```python
from build123d import *

# Parameters (mm, degrees)
SKETCH2_R           = 1.4
BOSS_EXTRUDE1_DEPTH = 2.5
SKETCH3_W           = 13
SKETCH3_H           = 4.686630076
BOSS_EXTRUDE3_DEPTH = 6
FILLET1_R           = 2
BOSS_EXTRUDE4_DEPTH = 0.5
CUT_EXTRUDE1_DEPTH  = 7


with BuildPart() as part:
    # Sketch1 → Revolve1 (revolve)
    with BuildSketch(Plane(origin=(0, 0, 0), x_dir=(0, 0, -1), z_dir=(1, 0, 0)), mode=Mode.PRIVATE) as revolve1_sk:
        Polygon((0, 0), (0, 11.5), (11, 11.5), (11, 4.5), (21, 4.5), (21, 3.175), (31, 3.175), (31, 0), align=None)
    revolve(revolve1_sk.sketch.rotate(Axis((0, 0, 0), (0, 0, -1)), 90), axis=Axis((0, 0, 0), (0, 0, -1)))

    # Sketch2 → Boss-Extrude1 (add)
    with BuildSketch(Plane(origin=(0, 0, -11), x_dir=(-1, 0, 0), z_dir=(0, 0, -1))):
        with Locations(Location((-10, 0, 0), (0, 0, 180))):
            Circle(SKETCH2_R)
    extrude(amount=BOSS_EXTRUDE1_DEPTH)

    # Sketch3 → Boss-Extrude3 (add)
    with BuildSketch(Plane(origin=(0, 0, -5), x_dir=(-1, 0, 0), z_dir=(0, 0, -1))):
        with Locations((0, -10.656684962)):
            Rectangle(SKETCH3_W, SKETCH3_H)
    extrude(amount=BOSS_EXTRUDE3_DEPTH)

    # Fillet1
    fillet1_edges = [part.edges().sort_by_distance(p)[0] for p in [
        (6.5, -9.486832981, -8),
        (-6.5, -9.486832981, -8),
    ]]
    fillet(fillet1_edges, radius=FILLET1_R)

    # Sketch4 → Boss-Extrude4 (add)
    # profile 1 of 3: a face of its own
    with BuildSketch(Plane(origin=(0, 0, -6), x_dir=(-1, 0, 0), z_dir=(0, 0, -1))):
        with BuildLine():
            Line((-5.420458078, -13), (-5.420458078, -13.616327338))
            Line((-5.420458078, -13.616327338), (-6, -13.616327338))
            Line((-6, -13.616327338), (-6, -15.080506085))
            Line((-6, -15.080506085), (-6.5, -15.080506085))
            Line((-6.5, -15.080506085), (-6.5, -18.5))
            ThreePointArc((-6.5, -18.5), (-5, -20), (-3.5, -18.5))
            Line((-3.5, -18.5), (-3.5, -15.080506085))
            Line((-3.5, -15.080506085), (-4, -15.080506085))
            Line((-4, -15.080506085), (-4, -13.616327338))
            Line((-4, -13.616327338), (-3.420458078, -13.616327338))
            Line((-3.420458078, -13.616327338), (-3.420458078, -13))
            Line((-3.420458078, -13), (-5.420458078, -13))
        make_face()
        with BuildLine():
            Line((-5.477176785, -18.5), (-5.477176785, -16.20237717))
            ThreePointArc((-5.477176785, -16.20237717), (-5, -15.725200384), (-4.522823215, -16.20237717))
            Line((-4.522823215, -16.20237717), (-4.522823215, -18.5))
            ThreePointArc((-4.522823215, -18.5), (-5, -18.977176785), (-5.477176785, -18.5))
        make_face(mode=Mode.SUBTRACT)
    # profile 2 of 3: a face of its own
    with BuildSketch(Plane(origin=(0, 0, -6), x_dir=(-1, 0, 0), z_dir=(0, 0, -1))):
        with BuildLine():
            Line((-1.5, -18.5), (-1.5, -15.080506085))
            Line((-1.5, -15.080506085), (-1, -15.080506085))
            Line((-1, -15.080506085), (-1, -13.616327338))
            Line((-1, -13.616327338), (-1.5, -13.616327338))
            Line((-1.5, -13.616327338), (-1.5, -13))
            Line((-1.5, -13), (1.5, -13))
            Line((1.5, -13), (1.5, -13.616327338))
            Line((1.5, -13.616327338), (1, -13.616327338))
            Line((1, -13.616327338), (1, -15.080506085))
            Line((1, -15.080506085), (1.5, -15.080506085))
            Line((1.5, -15.080506085), (1.5, -18.5))
            ThreePointArc((1.5, -18.5), (0, -20), (-1.5, -18.5))
        make_face()
        with BuildLine():
            Line((-0.477176785, -18.5), (-0.477176785, -16.20237717))
            ThreePointArc((-0.477176785, -16.20237717), (0, -15.725200384), (0.477176785, -16.20237717))
            Line((0.477176785, -16.20237717), (0.477176785, -18.5))
            ThreePointArc((0.477176785, -18.5), (0, -18.977176785), (-0.477176785, -18.5))
        make_face(mode=Mode.SUBTRACT)
    # profile 3 of 3: a face of its own
    with BuildSketch(Plane(origin=(0, 0, -6), x_dir=(-1, 0, 0), z_dir=(0, 0, -1))):
        with BuildLine():
            Line((3.420458078, -13.616327338), (3.420458078, -13))
            Line((3.420458078, -13), (5.420458078, -13))
            Line((5.420458078, -13), (5.420458078, -13.616327338))
            Line((5.420458078, -13.616327338), (6, -13.616327338))
            Line((6, -13.616327338), (6, -15.080506085))
            Line((6, -15.080506085), (6.5, -15.080506085))
            Line((6.5, -15.080506085), (6.5, -18.5))
            ThreePointArc((6.5, -18.5), (5, -20), (3.5, -18.5))
            Line((3.5, -18.5), (3.5, -15.080506085))
            Line((3.5, -15.080506085), (4, -15.080506085))
            Line((4, -15.080506085), (4, -13.616327338))
            Line((4, -13.616327338), (3.420458078, -13.616327338))
        make_face()
        with BuildLine():
            Line((4.522823215, -18.5), (4.522823215, -16.20237717))
            ThreePointArc((4.522823215, -16.20237717), (5, -15.725200384), (5.477176785, -16.20237717))
            Line((5.477176785, -16.20237717), (5.477176785, -18.5))
            ThreePointArc((5.477176785, -18.5), (5, -18.977176785), (4.522823215, -18.5))
        make_face(mode=Mode.SUBTRACT)
    extrude(amount=BOSS_EXTRUDE4_DEPTH)

    # Sketch5 → Cut-Extrude1 (cut)
    with BuildSketch(Plane(origin=(0, 0, -31), x_dir=(-1, 0, 0), z_dir=(0, 0, -1))):
        with BuildLine():
            Line((-2.740543661, 1.603136127), (2.740543661, 1.603136127))
            ThreePointArc((2.740543661, 1.603136127), (0, 3.175), (-2.740543661, 1.603136127))
        make_face()
    extrude(amount=-CUT_EXTRUDE1_DEPTH, mode=Mode.SUBTRACT)


solid = part.part
```
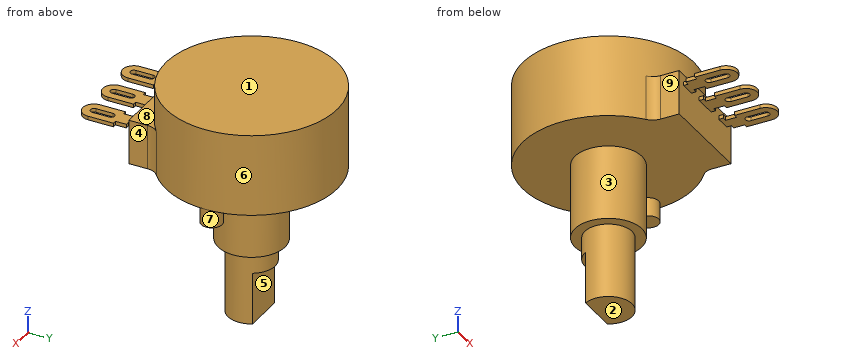
The listing builds one solid part. Answer for the finished solid, in the listing's coordinates (mm). Face numbers are marked on the shaded views. A direction names the side the tool comes from. Round coordinates to 2 decimals unless told otherwise and drop trailing zeros. Loops run counter-clockwise (first coordinate to the right, second up) from the corner with the lowest first, then second, coordinate; pieces in that order, holes last. Notation, with made-up numbers: (-22.75, 84.25) - (-2.75, 84.25) arc R11 ccw to (-2.75, 99.25) - close; hole circle Ø6 at (56, 47.25). An arc over 180 degrees is marked (long way). Return JSON: item names as keys, results as strings. Group by question number.
1. The part is cut by section A-A on x = 0. Determine the outline of the cut face in (y, z) (3 decimals).
2. Which of the six approach directions +Z, -Z, +X, -X, +Y, -Y give full straight-line access (tool end or side, diameter ignored) to the marked faces 1, 2, 3, 4 and 5?
3. Consider probe 1 along Z at (x, y) = (6, -1); probe 2 along Z at (x, y) = (-0.75, -12); probe 3 along X at (y, z) = (-4, -3.5). Determine where each line is inside the solid, lowest interval first.
4. The part is cut by section D-D on z = -15. Determine the outline of the cut face in (x, y).
5. The part is cut by section B-B on y = -14.5. Determine the outline of the cut face in (x, z), then the cut area to 3 significant figures.
6. Each of these flat-tipped pins is pushed along its axis until it touches: P1, Ø1.6, axis at x = 1, z = -28, coming from the +Y side; P2, Ø0.6, axis at y = -17, z = -6, coming from the +X side; P3, Ø3, axis at x = 4, y = 2, coming from the -Z side; P4, Ø0.9, axis at x = 5.5, y = -17, coming from the -Z side. Where does it stop, or does it pass through?
7. The part is cut by section C-C on y = 0. Determine the outline of the cut face in (x, z) (3 decimals), then the cut area to 4 significant figures.
8. The mould has two halves that part along X. Classify the marked faces 6, 7, 8 and 9: pulls with the +X half, pulls with the -X half, needs draft (parallel to the pull), parting line crosses it, or undercut.
Resolved:
{
 "1": {"outline": "(-20, -6.5) - (-18.977, -6.5) - (-18.977, -6) - (-20, -6) - close; (-15.725, -6.5) - (-13, -6.5) - (-13, -11) - (-4.5, -11) - (-4.5, -21) - (-3.175, -21) - (-3.175, -31) - (1.603, -31) - (1.603, -24) - (3.175, -24) - (3.175, -21) - (4.5, -21) - (4.5, -11) - (11.5, -11) - (11.5, 0) - (-11.5, 0) - (-11.5, -5) - (-13, -5) - (-13, -6) - (-15.725, -6) - close"},
 "2": {"face 1": "+Z, +X, -X, +Y, -Y", "face 2": "-Z, +X, -X, +Y, -Y", "face 3": "-Z", "face 4": "+Z, -Z, +X, -Y", "face 5": "-Z, +X, -X, +Y"},
 "3": {"probe 1": "z = -11 to 0", "probe 2": "z = -11 to -5", "probe 3": "x = -10.78 to 10.78"},
 "4": {"outline": "circle Ø9 at (0, 0)"},
 "5": {"outline": "(-6, -6.5) - (-4, -6.5) - (-4, -6) - (-6, -6) - close; (-1, -6.5) - (1, -6.5) - (1, -6) - (-1, -6) - close; (4, -6.5) - (6, -6.5) - (6, -6) - (4, -6) - close", "area": "3.00 mm²"},
 "6": {"P1": "stops at y = 1.6", "P2": "stops at x = 6.5", "P3": "stops at z = -31", "P4": "stops at z = -6.5"},
 "7": {"outline": "(-11.5, -11) - (-4.5, -11) - (-4.5, -21) - (-3.175, -21) - (-3.175, -31) - (3.175, -31) - (3.175, -21) - (4.5, -21) - (4.5, -11) - (8.6, -11) - (8.6, -13.5) - (11.4, -13.5) - (11.4, -11) - (11.5, -11) - (11.5, 0) - (-11.5, 0) - close", "area": "413.5 mm²"},
 "8": {"face 6": "parting line crosses it", "face 7": "undercut", "face 8": "needs draft", "face 9": "pulls with the -X half"}
}
